from build123d import *

# Parameters (mm, degrees)
F1_DEPTH = 38.1
F2_W     = 12.7
F2_H     = 12.7
F3_DEPTH = 5.08
F4_W     = 12.7
F4_H     = 25.4
F5_DEPTH = 12.7


with BuildPart() as f1:
    # F0 (on Front) → F1 (new body)
    with BuildSketch(Plane.XZ):
        Polygon((-77.360854, -0.949678), (-77.360854, -31.429678), (-26.560854, -31.429678), (-26.560854, -18.729678), (-64.660854, -18.729678), (-64.660854, -0.949678), align=None)
    extrude(amount=F1_DEPTH)

    # F2 (on face) → F3 (cut)
    with BuildSketch(Plane.XY.offset(-0.949678)):
        with Locations((-71.010854, -31.75)):
            Rectangle(F2_W, F2_H)
    extrude(amount=-F3_DEPTH, mode=Mode.SUBTRACT)

    # F4 (on face) → F5 (cut)
    with BuildSketch(Plane.XY.offset(-18.729678)):
        with Locations((-32.910854, -25.4)):
            Rectangle(F4_W, F4_H)
    extrude(amount=-F5_DEPTH, mode=Mode.SUBTRACT)


solid = f1.part
The listing builds one solid part. Answer for the finished solid, in the listing's coordinates (mm). A direction names the side the tool comes from. Round coordinates to 2 decimals unless told otherwise and drop trailing zeros. Write each loop counter-clockwise with the first axis right and the second up, starting at its lowest first coordinate (ties: lowest second). Pieces come first, ordered by that corner, then holes. Notation, with made-up numbers: (-24, -26) - (19, -26) arc R32 ccw to (19, 9) - close; hole circle Ø1 at (44.5, -3.75). An arc over 180 degrees is marked (long way). Use one line per item in the form item = value. Start each with the question number.
Item 1: Determine the mould class of faces 5 (the flat face through (-77.361, -19, -16)), 6 (the flat face through (-50, -19, -18.73)), 7 (the flat face through (-39.261, -26, -25)) for opening direction X: +X half, -X half, draft (parallel to the pull), parting line (faces both ways), or undercut.
Item 2: A cutting plane is placed at C-C (z = -4.5). Write down the section's boundary in (x, y).
Item 3: A tool of negligible diameter and unlimited length cuts with its end or side. For faces 1 (the flat face through (-71, -13, -0.95)), 2 (the flat face through (-71, -25.4, -3)), 3 (the flat face through (-33, -12.7, -25)), 4 (the flat face through (-64.661, -19, -10)), from which of +Z, -Z, +X, -X, +Y, -Y can it reach the whole face along a straight path? Write none if from no direction.
Item 4: A cutting plane is placed at D-D (x = -31.5). Write down the section's boundary in (y, z).
Item 5: Find the intervals of material crossed by line 1 (Z direction, x = -60, y = -29); line 2 (X direction, y = -13.5, z = -27); line 3 (X direction, y = -20, z = -10.5), in increasing order. Write a range as [from, to].
Item 6: A cutting plane is placed at B-B (y = -35.5). Write down the section's boundary in (x, z).
Item 7: A cutting plane is placed at A-A (x = -68). Write down the section's boundary in (y, z), plus the area to 3 significant figures.
Item 8: Flat-ended cylindrical pins translate along their axes: pin 1 Ø19 at (x, y) = (-41, -23.5) entering from +Z; pin 2 Ø10 at (y, z) = (-29.5, -26) entering from +X; pin 3 Ø2.5 at (x, z) = (-69, -4) entering from -Y; pin 4 Ø10 at (x, y) = (-33.5, -26.5) entering from +Z. Find the tip coordinate at first contact, or state that the pin passes through.
The answers:
q1.face_5 = -X half
q1.face_6 = draft
q1.face_7 = +X half
q2.outline = (-77.36, -25.4) - (-64.66, -25.4) - (-64.66, 0) - (-77.36, 0) - close
q3.face_1 = +Z, +X, -X, +Y, -Y
q3.face_2 = +Z, +X, -X, -Y
q3.face_3 = +Z, -Z, +X, -Y
q3.face_4 = +Z, +X, +Y, -Y
q4.outline = (-12.7, -31.43) - (0, -31.43) - (0, -18.73) - (-12.7, -18.73) - close
q5.line_1 = [-31.43, -18.73]
q5.line_2 = [-77.36, -39.26]
q5.line_3 = [-77.36, -64.66]
q6.outline = (-77.36, -31.43) - (-39.26, -31.43) - (-39.26, -18.73) - (-64.66, -18.73) - (-64.66, -6.03) - (-77.36, -6.03) - close
q7.outline = (-38.1, -31.43) - (0, -31.43) - (0, -0.95) - (-25.4, -0.95) - (-25.4, -6.03) - (-38.1, -6.03) - close
q7.area = 1,100 mm^2
q8.pin_1 = -18.73
q8.pin_2 = -39.26
q8.pin_3 = -25.4
q8.pin_4 = through
